Could you check a few things on this model? Use its own coordinates, in mm. A direction names the side the tool comes from. Round coordinates to 2 decimals unless told otherwise and drop trailing zeros. Loops run counter-clockwise (first coordinate to the right, second up) from the corner with the lowest first, then second, coordinate; pieces in that order, holes last. Notation, with made-up numbers: (52.25, -12) -> (83.25, -12) arc R11 cw to (83.25, 9) -> close; hole circle Ø7 at (-16, -17). An arc over 180 degrees is marked (long way). One line per item, written item: value.
```python
from build123d import *

# Parameters (mm, degrees)
SKETCH1_W           = 8.5
SKETCH1_H           = 8.5
BOSS_EXTRUDE1_DEPTH = 2
SKETCH2_R           = 4.05
SKETCH2_R_2         = 3.25
BOSS_EXTRUDE2_DEPTH = 2
SKETCH3_R           = 3.25
BOSS_EXTRUDE3_DEPTH = 4.3
SKETCH4_R           = 4.05
BOSS_EXTRUDE4_DEPTH = 1
SKETCH5_R           = 5.05
BOSS_EXTRUDE5_DEPTH = 2.5
SKETCH6_R           = 4.25
CUT_EXTRUDE1_DEPTH  = 0.2


with BuildPart() as part:
    # Sketch1 → Boss-Extrude1 (new body)
    with BuildSketch(Plane(origin=(0, 0, 0), x_dir=(1, 0, 0), z_dir=(0, 1, 0))):
        Rectangle(SKETCH1_W, SKETCH1_H)
    extrude(amount=BOSS_EXTRUDE1_DEPTH)

    # Sketch2 → Boss-Extrude2 (add)
    with BuildSketch(Plane(origin=(0, 2, 0), x_dir=(1, 0, 0), z_dir=(0, 1, 0))):
        with Locations(Location((0, 0, 0), (0, 0, 270))):
            Circle(SKETCH2_R)
        with Locations(Location((0, 0, 0), (0, 0, 270))):
            Circle(SKETCH2_R_2, mode=Mode.SUBTRACT)
    extrude(amount=BOSS_EXTRUDE2_DEPTH)

    # Sketch3 → Boss-Extrude3 (add)
    with BuildSketch(Plane(origin=(0, 2, 0), x_dir=(1, 0, 0), z_dir=(0, 1, 0))):
        with Locations(Location((0, 0, 0), (0, 0, 90))):
            Circle(SKETCH3_R)
    extrude(amount=BOSS_EXTRUDE3_DEPTH)

    # Sketch4 → Boss-Extrude4 (add)
    with BuildSketch(Plane(origin=(0, 6.3, 0), x_dir=(1, 0, 0), z_dir=(0, 1, 0))):
        with Locations(Location((0, 0, 0), (0, 0, 270))):
            Circle(SKETCH4_R)
    extrude(amount=BOSS_EXTRUDE4_DEPTH)

    # Sketch5 → Boss-Extrude5 (add)
    with BuildSketch(Plane(origin=(0, 7.3, 0), x_dir=(1, 0, 0), z_dir=(0, 1, 0))):
        with Locations(Location((0, 0, 0), (0, 0, 270))):
            Circle(SKETCH5_R)
    extrude(amount=BOSS_EXTRUDE5_DEPTH)

    # Sketch6 → Cut-Extrude1 (cut)
    with BuildSketch(Plane(origin=(0, 9.8, 0), x_dir=(1, 0, 0), z_dir=(0, 1, 0))):
        with Locations(Location((0, 0, 0), (0, 0, 270))):
            Circle(SKETCH6_R)
    extrude(amount=-CUT_EXTRUDE1_DEPTH, mode=Mode.SUBTRACT)


solid = part.part
```
Item 1: Will these pins go through, and if not, where does the flat tip stop? pin 1 Ø1 at (x, z) = (-1.5, -1) entering from +Y; pin 2 Ø1.6 at (x, y) = (-1.5, 1.5) entering from +Z; pin 3 Ø2 at (x, y) = (3.5, 4.5) entering from -Z.
Output:
pin 1: stops at y = 9.6
pin 2: stops at z = 4.25
pin 3: stops at z = -3.08
Item 2: If we section it at A-A on z = 0: List the corners of the cut face in (x, y) for me.
Output:
outline: (-5.05, 7.3) -> (-4.05, 7.3) -> (-4.05, 6.3) -> (-3.25, 6.3) -> (-3.25, 4) -> (-4.05, 4) -> (-4.05, 2) -> (-4.25, 2) -> (-4.25, 0) -> (4.25, 0) -> (4.25, 2) -> (4.05, 2) -> (4.05, 4) -> (3.25, 4) -> (3.25, 6.3) -> (4.05, 6.3) -> (4.05, 7.3) -> (5.05, 7.3) -> (5.05, 9.8) -> (4.25, 9.8) -> (4.25, 9.6) -> (-4.25, 9.6) -> (-4.25, 9.8) -> (-5.05, 9.8) -> close
Item 3: I need wall thicknesses on line 1 (X direction, y = 9.7, z = 0); line 2 (Y direction, x = 2.25, z = -4); line 3 (Y direction, x = 4, z = 1). Which ranges of each line are inside material? Lowest first, please. Write a range as from..to.
Output:
line 1: x = -5.05..-4.25, 4.25..5.05
line 2: y = 0..2, 7.3..9.8
line 3: y = 0..2, 7.3..9.6
Item 4: If we section it at C-C on z = 3.75: List the corners of the cut face in (x, y) for me, plus the area to 3 significant figures.
Output:
outline: (-4.25, 0) -> (4.25, 0) -> (4.25, 2) -> (1.53, 2) -> (1.53, 4) -> (-1.53, 4) -> (-1.53, 2) -> (-4.25, 2) -> close; (-3.38, 7.3) -> (-1.53, 7.3) -> (-1.53, 6.3) -> (1.53, 6.3) -> (1.53, 7.3) -> (3.38, 7.3) -> (3.38, 9.8) -> (2, 9.8) -> (2, 9.6) -> (-2, 9.6) -> (-2, 9.8) -> (-3.38, 9.8) -> close
area: 42.3 mm²
Item 5: If we section it at B-B on x = 3.75: List the corners of the cut face in (y, z) for me.
Output:
outline: (0, -4.25) -> (2, -4.25) -> (2, -1.53) -> (4, -1.53) -> (4, 1.53) -> (2, 1.53) -> (2, 4.25) -> (0, 4.25) -> close; (6.3, -1.53) -> (7.3, -1.53) -> (7.3, -3.38) -> (9.8, -3.38) -> (9.8, -2) -> (9.6, -2) -> (9.6, 2) -> (9.8, 2) -> (9.8, 3.38) -> (7.3, 3.38) -> (7.3, 1.53) -> (6.3, 1.53) -> close
Item 6: For faces 5 (the face through (-3.07, 8.53, -4.01)), 6 (the face through (-4, 9.8, -2)), 7 (the face through (-4.25, 1, 0)), 8 (the face through (-3, 2, -3)), 9 (the face through (4.25, 1, 0)), which set-ups out of +Z, -Z, +X, -X, +Y, -Y let a thin tool reach every point of the face, with its end or its side?
Output:
face 5: +Y
face 6: +Z, -Z, +X, -X, +Y
face 7: +Z, -Z, -X, -Y
face 8: none
face 9: +Z, -Z, +X, -Y
Item 7: If we section it at D-D on x = 0: List the corners of the cut face in (y, z) for me.
Output:
outline: (0, -4.25) -> (2, -4.25) -> (2, -4.05) -> (4, -4.05) -> (4, -3.25) -> (6.3, -3.25) -> (6.3, -4.05) -> (7.3, -4.05) -> (7.3, -5.05) -> (9.8, -5.05) -> (9.8, -4.25) -> (9.6, -4.25) -> (9.6, 4.25) -> (9.8, 4.25) -> (9.8, 5.05) -> (7.3, 5.05) -> (7.3, 4.05) -> (6.3, 4.05) -> (6.3, 3.25) -> (4, 3.25) -> (4, 4.05) -> (2, 4.05) -> (2, 4.25) -> (0, 4.25) -> close
Item 8: If we mould it in two halves opening along Z, with no side actions, what happens to faces 1 (the face through (-3.593, 6.793, 1.869)), 2 (the face through (0, 1, -4.25)), 3 (the face through (0, 1, 4.25)), 4 (the face through (0, 9.6, 0))? For each: released by +Z, released by -Z, zero draft, split by the parting line, or undercut.
Output:
face 1: split by the parting line
face 2: released by -Z
face 3: released by +Z
face 4: undercut
